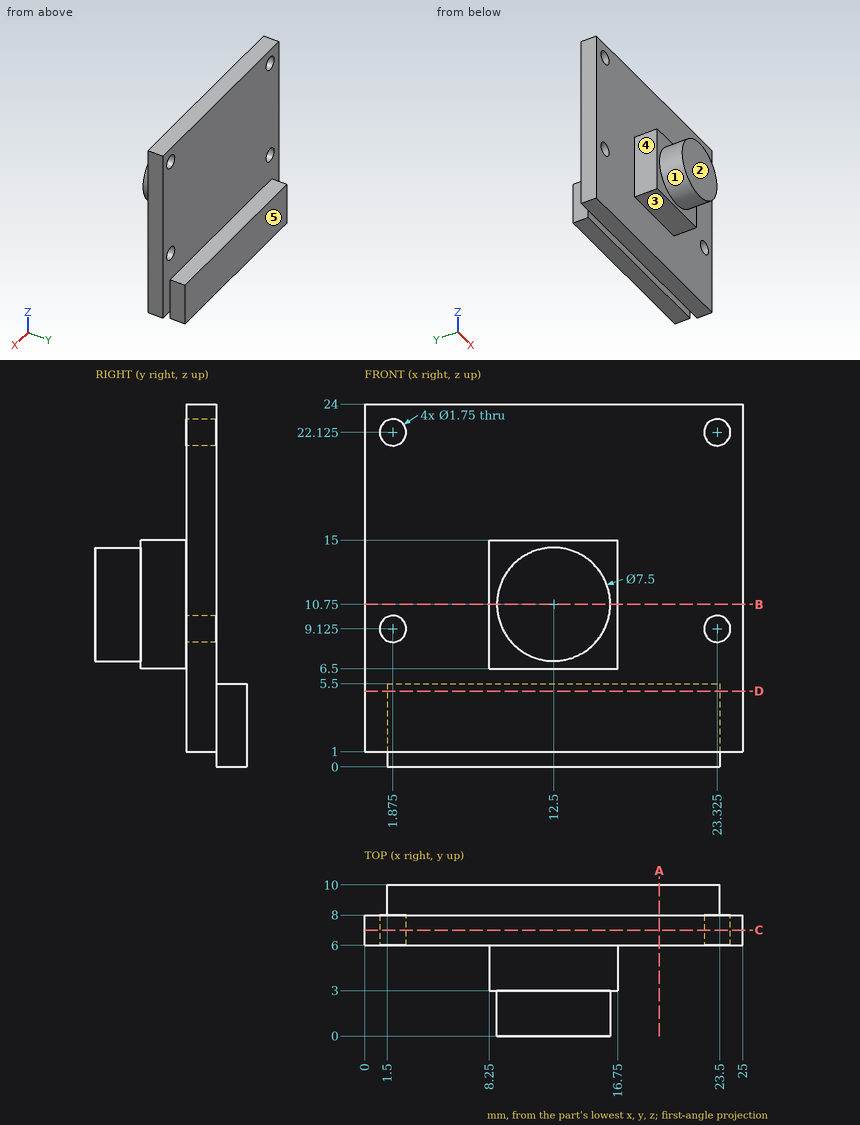
Design review of the part shown in the three views and the two pictorial views. Dimensions are in mm from the part's minimum x, y and z. A direction names the side the tool comes from. Coordinates: 2 decimals unless noted, no trailing zeros. Loops run counter-clockwise (first coordinate to the right, second up) from the corner with the lowest first, then second, coordinate; pieces in that order, holes last. Notation, with made-up numbers: (20, 3.5) -> (58, 3.5) arc R13 cw to (58, 13.5) -> close; hole circle Ø2 at (0.5, 8.25). An arc over 180 degrees is marked (long way). Answer as CSV lines item,"result".
Item 1: Insertion check: pin 1 (2 mm diameter, centred on x = 1.875, z = 9.125, fed in from -Y); pin 2 (1.5 mm diameter, centred on y = 4, z = 7.5, fed in from +X); pin 3 (11.5 mm diameter, centred on x = 18, z = 14, fed in from +Y). Each pin has a flat end and moves straight along its axis. Give the tip position at first contact, or say it passes through.
Results below:
pin 1,"stops at y = 6"
pin 2,"stops at x = 16.75"
pin 3,"stops at y = 8"
Item 2: Machinability: for the marked faces 1, 2, 3, 4 and 5, which of the approach directions +Z, -Z, +X, -X, +Y, -Y give a long, thin tool a straight path to every point of the face, cutting with its end or side? Answer none if there is none.
Results below:
face 1,"-Y"
face 2,"+Z, -Z, +X, -X, -Y"
face 3,"-Z, +X, -X, -Y"
face 4,"+Z, -Z, -X, -Y"
face 5,"+Z, -Z, +X, -X, +Y"
Item 3: Take a section at C-C, the plane y = 7. State the section outline as (x, z) points (3 decimals), and give its area (3 significant figures).
Results below:
outline,"(0, 1) -> (25, 1) -> (25, 24) -> (0, 24) -> close; hole circle Ø1.75 at (1.875, 9.125); hole circle Ø1.75 at (1.875, 22.125); hole circle Ø1.75 at (23.325, 9.125); hole circle Ø1.75 at (23.325, 22.125)"
area,"565 mm2"
Item 4: Take a section at D-D, the plane z = 5. State the section outline as (x, y) points, and give its area (3 significant figures).
Results below:
outline,"(0, 6) -> (25, 6) -> (25, 8) -> (23.5, 8) -> (23.5, 10) -> (1.5, 10) -> (1.5, 8) -> (0, 8) -> close"
area,"94.0 mm2"
Item 5: Take a section at B-B, the plane z = 10.75. State the section outline as (x, y) points, and give its area (3 significant figures).
Results below:
outline,"(0, 6) -> (8.25, 6) -> (8.25, 3) -> (8.75, 3) -> (8.75, 0) -> (16.25, 0) -> (16.25, 3) -> (16.75, 3) -> (16.75, 6) -> (25, 6) -> (25, 8) -> (0, 8) -> close"
area,"98.0 mm2"
Item 6: Take a section at A-A, the plane x = 19.5. State the section outline as (y, z) points.
Results below:
outline,"(6, 1) -> (8, 1) -> (8, 0) -> (10, 0) -> (10, 5.5) -> (8, 5.5) -> (8, 24) -> (6, 24) -> close"
Item 7: For L1, parallel to Z at x = 18.5, y = 9; L2, parallel to Y at x = 19.75, z = 15; L3, parallel to X at y = 5.5, z = 10, list the stretches that pass through material, from the lowest coordinate up.
Results below:
L1,"z = 0 to 5.5"
L2,"y = 6 to 8"
L3,"x = 8.25 to 16.75"
